The listing builds one solid part. Answer for the finished solid, in the listing's coordinates (mm). Round coordinates to 2 decimals unless told otherwise and drop trailing zeros. Write each loop counter-clockwise with the first axis right and the second up, starting at its lowest first coordinate (ties: lowest second). Pieces come first, ordered by that corner, then holes. Notation, with made-up numbers: (8.5, -7) - (15.5, -7) arc R26 ccw to (15.5, 29) - close; hole circle Ø7 at (51.25, -21). An arc over 180 degrees is marked (long way). Answer as CSV lines item,"result". Start each with the question number.
Item 1: Straight lines are drawn through the part: line 1 along Z through (x, y) = (36.5, 11.5); line 2 along Z through (x, y) = (6.5, 4.5); line 3 along X through (y, z) = (47.5, 30) (3 decimals). For each, find the intervals that lie inside material, in ascending order. Write a range as [from, to].
Item 2: A cutting plane is placed at B-B on z = -386. Determine the outline of the cut face in (x, y), and give its area (3 significant figures).
Item 3: A cutting plane is placed at A-A on x = 54. Determine the outline of the cut face in (y, z).
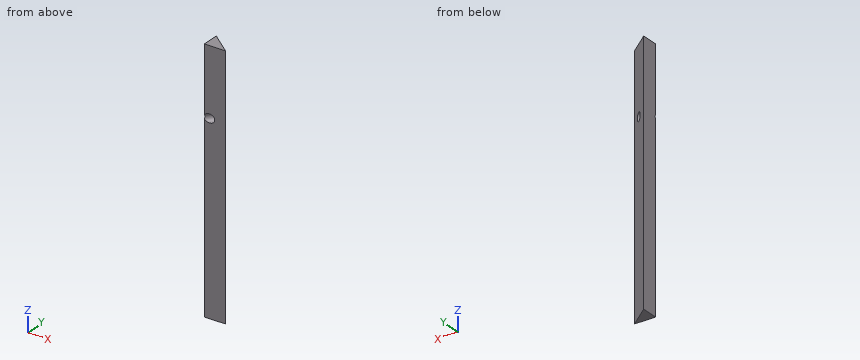
```python
from build123d import *

# Parameters (mm, degrees)
BOSS_EXTRUDE1_DEPTH = 38.1
BOSS_EXTRUDE2_DEPTH = 292.1
BOSS_EXTRUDE3_DEPTH = 431.8
SKETCH6_R           = 12.7
CUT_EXTRUDE2_DEPTH  = 431.8


with BuildPart() as part:
    # Sketch1 → Boss-Extrude1 (new body)
    with BuildSketch(Plane.XY):
        Polygon((0, 0), (0, 50.8), (63.5, 0), align=None)
    extrude(amount=-BOSS_EXTRUDE1_DEPTH)

    # Sketch3 → Boss-Extrude2 (add)
    with BuildSketch(Plane.XY):
        Polygon((0, 50.8), (0, 0), (63.5, 0), align=None)
    extrude(amount=BOSS_EXTRUDE2_DEPTH)

    # Sketch4 → Boss-Extrude3 (add)
    with BuildSketch(Plane(origin=(0, 0, -38.1), x_dir=(-1, 0, 0), z_dir=(0, 0, -1))):
        Polygon((0, 50.8), (-63.5, 0), (0, 0), align=None)
    extrude(amount=BOSS_EXTRUDE3_DEPTH)

    # Sketch6 → Cut-Extrude2 (cut)
    with BuildSketch(Plane(origin=(24.780487805, 30.975609756, 0), x_dir=(0.780868809, -0.624695048, 0), z_dir=(0.624695048, 0.780868809, 0))):
        with Locations((11.4851694, -88.9)):
            Circle(SKETCH6_R)
    extrude(amount=-CUT_EXTRUDE2_DEPTH, mode=Mode.SUBTRACT)


solid = part.part
```
Geometry says:
1,line 1,"z = [-469.9, 80.86], [96.94, 292.1]"
1,line 2,"z = [-469.9, 80.17], [97.63, 292.1]"
1,line 3,"x = [0, 4.125]"
2,outline,"(0, 0) - (63.5, 0) - (0, 50.8) - close"
2,area,"1,610 mm^2"
3,outline,"(0, -469.9) - (7.6, -469.9) - (7.6, 292.1) - (0, 292.1) - close"
